```python
from build123d import *

# Parameters (mm, degrees)
F1_DEPTH = 39
F2_W     = 3
F2_H     = 4.5
F3_DEPTH = 0.5
F4_W     = 3.197795
F4_H     = 4.5
F5_DEPTH = 1


with BuildPart() as f1:
    # F0 (on Top) → F1 (new body)
    with BuildSketch(Plane.XY):
        Polygon((-3, 0.603), (0.5, 0.603), (0.5, 6), (30, 33.67), (33, 33.67), (33, 34.17), (29.802205, 34.17), (0, 6.216542), (0, 1.103), (-3, 1.103), align=None)
    extrude(amount=F1_DEPTH)

    # F2 (on face) → F3 (cut, through all)
    with BuildSketch(Plane(origin=(0, 1.103, 0), x_dir=(-1, 0, 0), z_dir=(0, 1, 0))):
        with Locations((1.5, 2.25)):
            Rectangle(F2_W, F2_H)
        with Locations((1.5, 36.75)):
            Rectangle(F2_W, F2_H)
    extrude(amount=-F3_DEPTH, mode=Mode.SUBTRACT)

    # F4 (on face) → F5 (cut)
    with BuildSketch(Plane(origin=(0, 34.17, 0), x_dir=(-1, 0, 0), z_dir=(0, 1, 0))):
        with Locations((-31.401103, 36.75)):
            Rectangle(F4_W, F4_H)
        with Locations((-31.401103, 2.25)):
            Rectangle(F4_W, F4_H)
    extrude(amount=-F5_DEPTH, mode=Mode.SUBTRACT)


solid = f1.part
```
Build history of the part. All positions in model axes, mm. A direction names the side the tool comes from. Coordinates: 2 decimals unless noted, no trailing zeros. Order: outer loops, then holes, each group sorted by start corner. A loop starts at its lowest first (then second) coordinate and runs counter-clockwise, first axis right, second up.
Item 1: Saw through at B-B on y = 5. List the corners of the cut face in (x, z).
Filled in:
outline: (0, 0) - (0.5, 0) - (0.5, 39) - (0, 39) - close
Item 2: Saw through at C-C on x = -1. List the corners of the cut face in (y, z).
Filled in:
outline: (0.6, 4.5) - (1.1, 4.5) - (1.1, 34.5) - (0.6, 34.5) - close
Item 3: Saw through at A-A on z = 30. List the corners of the cut face in (x, y), then the cut area to 3 significant figures.
Filled in:
outline: (-3, 0.6) - (0.5, 0.6) - (0.5, 6) - (30, 33.67) - (33, 33.67) - (33, 34.17) - (29.8, 34.17) - (0, 6.22) - (0, 1.1) - (-3, 1.1) - close
area: 26.1 mm2
Item 4: Tool access for faces 1 (the flat face through (31, 33.67, 19)), 2 (the flat face through (-1, 1.103, 19)), 3 (the flat face through (-1, 0.603, 19)): list every direction of +Z, -Z, +X, -X, +Y, -Y with a clear straight run to the whole face (end or side of a thin tool).
Filled in:
face 1: +Z, -Z, +X, -Y
face 2: +Z, -Z, -X, +Y
face 3: +Z, -Z, +X, -X, -Y
Item 5: Drill centre lines: L1, parallel to Y at x = 30.5, z = 26; L2, parallel to X at y = 2.5, z = 2.5; L3, parallel to Y at x = 4.5, z = 5. Where is each one in solid material? Low to high.
Filled in:
L1: y = 33.67 to 34.17
L2: x = 0 to 0.5
L3: y = 9.75 to 10.44
Item 6: Drop flat-ended pins along their axis: pin 1 Ø1 at (y, z) = (13, 28.5) entering from -X; pin 2 Ø0.5 at (x, y) = (31.5, 34) entering from +Z; pin 3 Ø10 at (x, z) = (13, 21.5) entering from +Y. Give the stop position or say it passes through.
Filled in:
pin 1: stops at x = 6.7
pin 2: stops at z = 34.5
pin 3: stops at y = 23.1
